Source: CAD feature listing. Evaluate the final solid. Frame: model axes, mm. Face numbers are marked on the shaded views. A direction names the side the tool comes from. Coordinates: 2 decimals unless noted, no trailing zeros. Loops run counter-clockwise (first coordinate to the right, second up) from the corner with the lowest first, then second, coordinate; pieces in that order, holes last.
Autodesk Inventor part; units mm, degrees
ref_plane "YZ Plane" through (0, 0, 0) normal (1, 0, 0) x (0, 1, 0)
ref_plane "XZ Plane" through (0, 0, 0) normal (0, 1, 0) x (-1, 0, 0)
ref_plane "XY Plane" through (0, 0, 0) normal (0, 0, 1) x (1, 0, 0)
sketch "Boceto1" plane through (0, 0, 0) normal (0, 0, 1) x (1, 0, 0)
  line L0 (0, 0) -> (35, 0)
  line L1 (35, 0) -> (35, 10)
  line L2 (35, 10) -> (0, 10)
  line L3 (0, 10) -> (0, 0)
  dimension "d0" = 35
  dimension "d1" = 10
extrude "Extrusión1" add sketch "Boceto1" along normal blind 40
sketch "Boceto2" plane through (0, 0, 40) normal (0, 0, 1) x (1, 0, 0)
  line L0 (35, 0) -> (35, 10) construction
  line L1 (35, 10) -> (0, 10) construction
  line L2 (0, 10) -> (0, 0) construction
  line L3 (0, 0) -> (35, 0) construction
  line L4 (35, 10) -> (0, 10)
  line L5 (0, 0) -> (35, 0)
  line L6 (6, 10) -> (29, 10)
  line L7 (29, 10) -> (29, 0)
  line L8 (29, 0) -> (6, 0)
  line L9 (6, 0) -> (6, 10)
  line L10 (17.5, 10) -> (17.5, 0) construction
  dimension "d4" = 23
  dimension "d5" = 11.5
extrude "Extrusión2" cut sketch "Boceto2" against normal blind 13
sketch "Boceto3" plane through (0, 0, 0) normal (0, 0, -1) x (-1, 0, 0)
  line L0 (-35, 0) -> (-35, 10) construction
  line L1 (0, 0) -> (-35, 0) construction
  line L2 (0, 10) -> (0, 0) construction
  line L3 (-35, 10) -> (0, 10) construction
  line L4 (-35, 10) -> (-45, 10)
  line L5 (-45, 10) -> (-45, 0)
  line L6 (-45, 0) -> (-35, 0)
  line L7 (-35, 0) -> (-35, 10)
  line L8 (-6, 10) -> (0, 10)
  line L9 (0, 10) -> (10, 10)
  line L10 (10, 10) -> (10, 0)
  line L11 (10, 0) -> (0, 0)
  line L12 (0, 0) -> (0, 10)
  line L13 (-35, 0) -> (-35, 10) construction
  line L14 (0, 10) -> (0, 0) construction
  dimension "d8" = 10
  dimension "d9" = 10
extrude "Extrusión3" add sketch "Boceto3" against normal blind 3
fillet "Empalme1" radius 4 8 edges at (-10, 0, 1.5) (-10, 10, 1.5) (45, 0, 1.5) (45, 10, 1.5) (0, 5, 40) (35, 5, 40) (0, 5, 3) (35, 5, 3)
sketch "Boceto5" plane through (0, 0, 3) normal (0, 0, 1) x (1, 0, 0)
  line L0 (-4, 10) -> (-4, 0) construction
  line L1 (-4, 10) -> (-6, 10) construction
  arc A0 (-6, 10) -> (-10, 6) centre (-6, 6) ccw construction
  line L2 (-10, 6) -> (-10, 4) construction
  arc A1 (-10, 4) -> (-6, 0) centre (-6, 4) ccw construction
  line L3 (-6, 0) -> (-4, 0) construction
  line L4 (39, 0) -> (39, 10) construction
  line L5 (39, 0) -> (41, 0) construction
  arc A2 (41, 0) -> (45, 4) centre (41, 4) ccw construction
  line L6 (45, 4) -> (45, 6) construction
  arc A3 (45, 6) -> (41, 10) centre (41, 6) ccw construction
  line L7 (41, 10) -> (39, 10) construction
  line L8 (-10, 5) -> (45, 5) construction
  circle A4 centre (-6.5, 5) radius 1.6
  circle A5 centre (41.5, 5) radius 1.6
  point P0 (0, 0)
  dimension "d15" = 3.2
  dimension "d16" = 3.2
  dimension "d17" = 3.5
  dimension "d18" = 3.5
extrude "Extrusión4" cut sketch "Boceto5" against normal blind 10
chamfer "Chaflán1" distance 0.5 angle 45 28 edges at (-8.8284, 1.1716, 3) (-10, 5, 3) (-8.8284, 8.8284, 3) (-5, 10, 3) (0, 10, 21.5) (1.1716, 10, 38.8284) (5, 10, 40) (-5, 0, 3) (0, 0, 21.5) (1.1716, 0, 38.8284) (5, 0, 40) (40, 0, 3) (43.8284, 1.1716, 3) (45, 5, 3) (43.8284, 8.8284, 3) (40, 10, 3) (35, 10, 21.5) (33.8284, 10, 38.8284) (30, 10, 40) (35, 0, 21.5) (33.8284, 0, 38.8284) (30, 0, 40) (6, 5, 40) (29, 5, 40) (6, 0, 33.5) (6, 10, 33.5) (29, 0, 33.5) (29, 10, 33.5)
sketch "Boceto6" plane through (-6, 0, 0) normal (0, -1, 0) x (1, 0, 0)
  line L0 (45, 2.5) -> (47, 2.5) construction
  arc A0 (40.5, 7) -> (45, 2.5) centre (45, 7) ccw construction
  line L1 (40.5, 36) -> (40.5, 7) construction
  arc A1 (40.5, 36) -> (37, 39.5) centre (37, 36) ccw construction
  line L2 (35.5, 39.5) -> (37, 39.5) construction
  line L3 (35.5, 27) -> (35.5, 39.5) construction
  line L4 (35.5, 27) -> (11.5, 27) construction
  line L5 (11.5, 39.5) -> (11.5, 27) construction
  line L6 (10, 39.5) -> (11.5, 39.5) construction
  arc A2 (10, 39.5) -> (6.5, 36) centre (10, 36) ccw construction
  line L7 (6.5, 7) -> (6.5, 36) construction
  arc A3 (2, 2.5) -> (6.5, 7) centre (2, 7) ccw construction
  line L8 (0, 2.5) -> (2, 2.5) construction
  line L9 (0, 0) -> (0, 2.5) construction
  line L10 (47, 0) -> (0, 0) construction
  line L11 (47, 2.5) -> (47, 0) construction
  arc A4 (10, 39.5) -> (6.5, 36) centre (10, 36) ccw construction
  line L12 (9.5, 39.4641) -> (9.5, 0) construction
  line L13 (47, 0) -> (0, 0) construction
  arc A5 (40.5, 36) -> (37, 39.5) centre (37, 36) ccw construction
  line L14 (37.5, 39.4641) -> (37.5, 0) construction
  line L15 (23.5, 0) -> (23.5, 27) construction
  line L16 (6.5, 33.2) -> (40.5, 33.2) construction
  line L17 (40.5, 7) -> (40.5, 36) construction
  circle A6 centre (9.5, 33.2) radius 1.75
  circle A7 centre (37.5, 33.2) radius 1.75
  point P0 (6, 0)
  dimension "d26" = 28
  dimension "d27" = 14
  dimension "d28" = 6.2
  dimension "d29" = 3.5
  dimension "d30" = 3.5
extrude "Extrusión5" cut sketch "Boceto6" against normal blind 5
equation "\"d5\" = 0.5 * d4"
equation "\"d27\" = 0.5 * d26"
properties part number "base_servo"
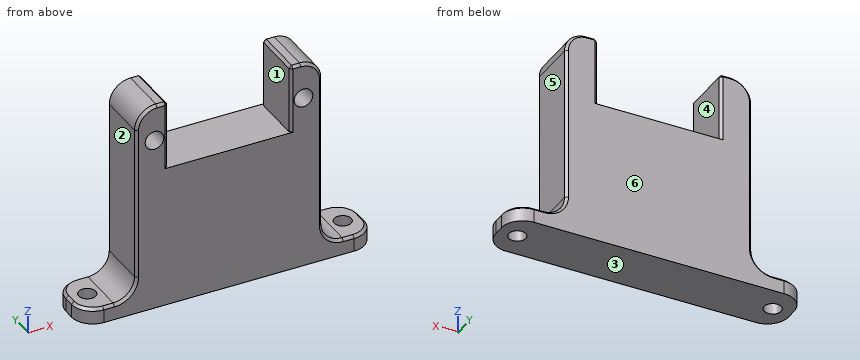
Q1. Contact query for flat-ended pins moving along their axis: pin 1 Ø6 at (y, z) = (2, 17) entering from +X; pin 2 Ø5 at (y, z) = (3.5, 23) entering from -X; pin 3 Ø3 at (x, y) = (42, 6) entering from +Z. Output: stop coordinate, or through.
Q2. Section B-B, the plane z = 10. Return the cut outline in (x, y), plus the area to 4 significant figures.
Q3. Section C-C, the plane x = 15.5. Return the cut outline in (y, z).
Q4. Line query: line 1 along X through (y, z) = (8.5, 33.5); line 2 along X through (y, z) = (9, 21); line 3 along Z through (x, y) = (22, 2.5). Output: solid intervals per line, ascending.
Q5. Draft query along X for the marked faces 1, 2 and 3. Return one class per face: +X half, -X half, draft (parallel to the pull), parting line (faces both ways), or undercut.
Q6. Section D-D, the plane z = 33.2. Return the cut outline in (x, y), plus the area to 3 significant figures.
Q7. Section A-A, the plane z = 29. Return the cut outline in (x, y), plus the area to 3 significant figures.
Q8. Access query for the marked faces 4, 5 and 6. Directions: +Z, -Z, +X, -X, +Y, -Y. A direction counts if a zero-diameter tool reaches every point of the face in a straight line with its end or side. Return the directions, or none.
Derived:
1. pin 1: stops at x = 35
1. pin 2: stops at x = 0
1. pin 3: stops at z = 3
2. outline: (0, 0.5) - (0.5, 0) - (34.5, 0) - (35, 0.5) - (35, 9.5) - (34.5, 10) - (0.5, 10) - (0, 9.5) - close
2. area: 349.5 mm2
3. outline: (0, 0) - (10, 0) - (10, 27) - (0, 27) - close
4. line 1: x = 0 to 6, 29 to 35
4. line 2: x = 0 to 35
4. line 3: z = 0 to 27
5. face 1: undercut
5. face 2: -X half
5. face 3: draft
6. outline: (0, 0.5) - (0.5, 0) - (1.75, 0) - (1.75, 5) - (5.25, 5) - (5.25, 0) - (5.5, 0) - (6, 0.5) - (6, 9.5) - (5.5, 10) - (0.5, 10) - (0, 9.5) - close; (29, 0.5) - (29.5, 0) - (29.75, 0) - (29.75, 5) - (33.25, 5) - (33.25, 0) - (34.5, 0) - (35, 0.5) - (35, 9.5) - (34.5, 10) - (29.5, 10) - (29, 9.5) - close
6. area: 84.0 mm2
7. outline: (0, 0.5) - (0.5, 0) - (5.5, 0) - (6, 0.5) - (6, 9.5) - (5.5, 10) - (0.5, 10) - (0, 9.5) - close; (29, 0.5) - (29.5, 0) - (34.5, 0) - (35, 0.5) - (35, 9.5) - (34.5, 10) - (29.5, 10) - (29, 9.5) - close
7. area: 119 mm2
8. face 4: +Z, +Y, -Y
8. face 5: +Z, +X, +Y, -Y
8. face 6: +Z, -Z, +X, -X, +Y
